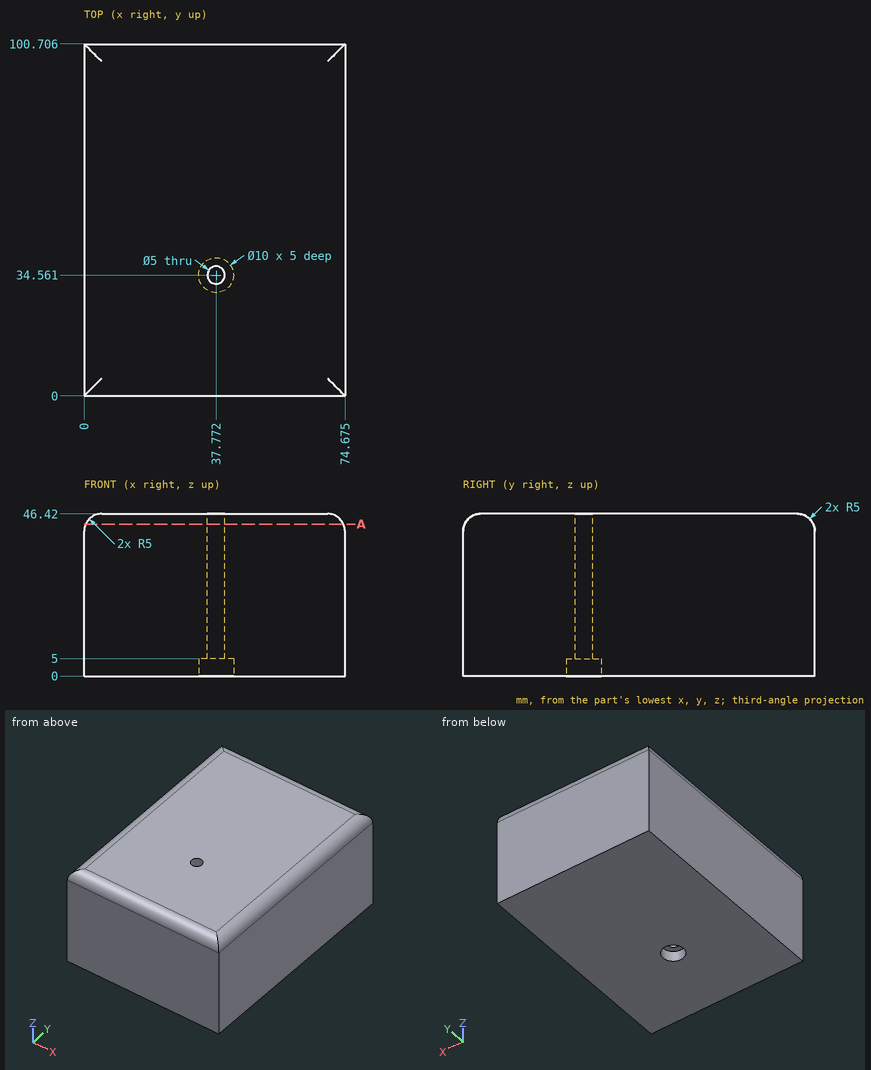
The figure shows three views and two pictorial views of one solid part (mm, origin at its lowest corner). Answer the questions. Coordinates: 2 decimals unless noted, no trailing zeros. Loops run counter-clockwise (first coordinate to the right, second up) from the corner with the lowest first, then second, coordinate; pieces in that order, holes last. Notation, with made-up numbers: (-23.75, -3.5) -> (6.25, -3.5) arc R22 cw to (6.25, 35.5) -> close; hole circle Ø7 at (77, -8). An arc over 180 degrees is marked (long way). Use one line per item in the form item = value. Start each with the question number.
Item 1: A flat-ended cylindrical pin translates along its axis: pin 1 Ø9 at (x, y) = (37.77, 34.56) entering from -Z. Find the tip coordinate at first contact, or state that the pin passes through.
Item 2: Consider L1, parallel to Y at x = 39.5, z = 17 (1 decimal); L2, parallel to Z at x = 20, y = 4; L3, parallel to X at y = 80, z = 44 (1 decimal). Determine where each line is inside the solid, lowest interval first. Write a range as [from, to].
Item 3: The part is cut by section A-A on z = 43.5. Determine the outline of the cut face in (x, y).
Answer key:
q1.pin_1 = 5
q2.L1 = [0, 32.8], [36.4, 100.7]
q2.L2 = [0, 46.32]
q2.L3 = [0.7, 74]
q3.outline = (0.45, 0.45) -> (74.22, 0.45) -> (74.22, 100.25) -> (0.45, 100.25) -> close; hole circle Ø5 at (37.77, 34.56)
